Build history of the part. All positions in model axes, mm. Face numbers are marked on the shaded views. A direction names the side the tool comes from. Give positions to 0.01 mm unless a question says otherwise; leave off trailing zeros. Loops run counter-clockwise (first coordinate to the right, second up) from the corner with the lowest first, then second, coordinate; pieces in that order, holes last.
1) Wall check: line 1 (Y direction, x = 2.5, z = 0); line 2 (Z direction, x = 5.65, y = 3.5); line 3 (Y direction, x = 4.7, z = 21.5). Give the ranges that are in metal, low to high.
2) 3-axis set-ups, long thin cutter, end or side, ignore diameter. For the marked faces 4 and 5: which of +Z, -Z, +X, -X, +Y, -Y reach the whole face in a straight line?
3) Two-plate mould, pull along Z, no slides. Class the marked faces 1, 2 and 3: +Z half, -Z half, draft (parallel to the pull), parting line (faces both ways), or undercut.
4) Flat gauge pins, fed straight in: P1, Ø1.4, axis at y = 4, z = -31.5, coming from the +X side; P2, Ø11.5, axis at y = 63, z = 0, coming from the +X side. Where does each tip first touch, or does it go through?
5) Band-saw the part on A-A on y = 4. List the corners of the cut face in (x, z).
6) Band-saw the part on D-D on z = -31.5. List the corners of the cut face in (x, y), then the cut area to 3 significant figures.
7) Band-saw the part on C-C on x = 4.05. State how many separate pieces and enclosed holes the cut face has, then the cut area to 3 significant figures.
8) Band-saw the part on B-B on z = -21.5. List the corners of the cut face in (x, y).
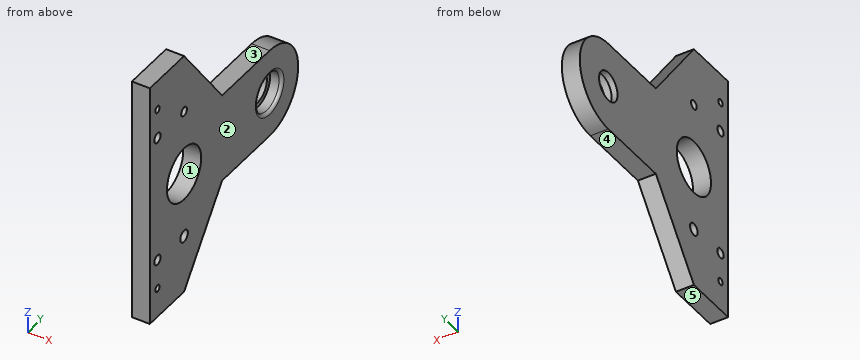
Autodesk Inventor part; units mm, degrees
ref_plane "YZ Plane" through (0, 0, 0) normal (1, 0, 0) x (0, 1, 0)
ref_plane "XZ Plane" through (0, 0, 0) normal (0, 1, 0) x (-1, 0, 0)
ref_plane "XY Plane" through (0, 0, 0) normal (0, 0, 1) x (1, 0, 0)
sketch "스케치1" plane through (0, 0, 0) normal (1, 0, 0) x (0, 1, 0)
  line L0 (0, -41.5) -> (18, -41.5)
  line L1 (18, -41.5) -> (18, 59.6584) construction
  line L2 (0, 0) -> (0, -41.5)
  line L3 (84.3904, 0) -> (-15.1692, 0) construction
  arc A0 (63, -15) -> (78, 0) centre (63, 0) ccw
  line L4 (63, -15) -> (38, -15)
  line L5 (38, -15) -> (18, -41.5)
  line L6 (0, 41.5) -> (18, 41.5)
  line L7 (0, 0) -> (0, 41.5)
  arc A1 (78, 0) -> (63, 15) centre (63, 0) ccw
  line L8 (63, 15) -> (38, 15)
  line L9 (38, 15) -> (18, 41.5)
  dimension "d0" = 18
  dimension "d8" = 45
  dimension "d9" = 25
extrude "돌출1" add sketch "스케치1" along normal blind 6
sketch "스케치2" plane through (6, 0, 0) normal (1, 0, 0) x (0, 0, -1)
  line L0 (-58.8675, 4) -> (65.7315, 4) construction
  line L1 (-41.5, 0) -> (41.5, 0)
  circle A0 centre (31.5, 4) radius 1.15
  circle A1 centre (21.5, 4) radius 1.65
  line L2 (41.5, 0) -> (41.5, 18)
  line L3 (0, 13.8041) -> (0, -7.7982) construction
  circle A2 centre (-31.5, 4) radius 1.15
  circle A3 centre (-21.5, 4) radius 1.65
  point P0 (0, 0)
  dimension "d12" = 4
  dimension "d13" = 2.3
  dimension "d14" = 3.3
  dimension "d15" = 10
  dimension "d16" = 20
  dimension "d32" = 21.5
extrude "돌출2" cut sketch "스케치2" against normal blind 6
sketch "스케치3" plane through (6, 0, 0) normal (1, 0, 0) x (0, 0, -1)
  line L0 (-41.5, 18) -> (-41.5, 0)
  line L1 (41.5, 0) -> (41.5, 18)
  line L2 (-41.5, 18) -> (41.5, 18) construction
  line L3 (-21.915, 37.5775) -> (-21.915, 10.4705) construction
  line L4 (0, 43.7434) -> (0, -15.8221) construction
  line L5 (21.915, 37.5775) -> (21.915, 10.4705) construction
  circle A0 centre (-21.915, 18) radius 1.5
  circle A1 centre (21.915, 18) radius 2
  circle A2 centre (0, 18) radius 9
  point P0 (0, 0)
  dimension "d19" = 21.915
  dimension "d20" = 3
  dimension "d21" = 4
  dimension "d22" = 18
extrude "돌출3" cut sketch "스케치3" against normal blind 6
sketch "스케치4" plane through (6, 0, 0) normal (1, 0, 0) x (0, 0, -1)
  arc A0 (15, 63) -> (-15, 63) centre (0, 63) ccw
  circle A1 centre (0, 63) radius 6.5
  point P0 (0, 0)
  dimension "d25" = 13
extrude "돌출4" cut sketch "스케치4" against normal blind 4
sketch "스케치5" plane through (2, 63, 0) normal (1, 0, 0) x (0, 0, -1)
  circle A0 centre (0, 0) radius 4.85
  point P0 (0, -63)
  dimension "d28" = 9.7
extrude "돌출5" cut sketch "스케치5" against normal blind 2
fillet "모깎기1" radius 1 1 edges at (6, 63, 6.5)
properties part number "탑(모터쪽옆면수정)"
Findings below:
1. line 1: y = 0 to 9, 27 to 56.5, 69.5 to 78
1. line 2: z = -41.5 to -32.54, -30.46 to -23.07, -19.93 to 19.93, 23.07 to 30.46, 32.54 to 41.5
1. line 3: y = 0 to 2.35, 5.65 to 16.56, 19.44 to 33.09
2. face 4: -Z, +X, -X, +Y
2. face 5: -Z, +X, -X, +Y, -Y
3. face 1: undercut
3. face 2: draft
3. face 3: +Z half
4. P1: passes through
4. P2: stops at x = 2
5. outline: (0, -41.5) - (6, -41.5) - (6, -32.65) - (0, -32.65) - close; (0, -30.35) - (6, -30.35) - (6, -23.15) - (0, -23.15) - close; (0, -19.85) - (6, -19.85) - (6, 19.85) - (0, 19.85) - close; (0, 23.15) - (6, 23.15) - (6, 30.35) - (0, 30.35) - close; (0, 32.65) - (6, 32.65) - (6, 41.5) - (0, 41.5) - close
6. outline: (0, 0) - (6, 0) - (6, 2.85) - (0, 2.85) - close; (0, 5.15) - (6, 5.15) - (6, 25.55) - (0, 25.55) - close
6. area: 139 mm2
7. separate pieces: 1
7. enclosed holes: 8
7. area: 3,300 mm2
8. outline: (0, 0) - (6, 0) - (6, 2.35) - (0, 2.35) - close; (0, 5.65) - (6, 5.65) - (6, 16.04) - (0, 16.04) - close; (0, 19.96) - (6, 19.96) - (6, 33.09) - (0, 33.09) - close
